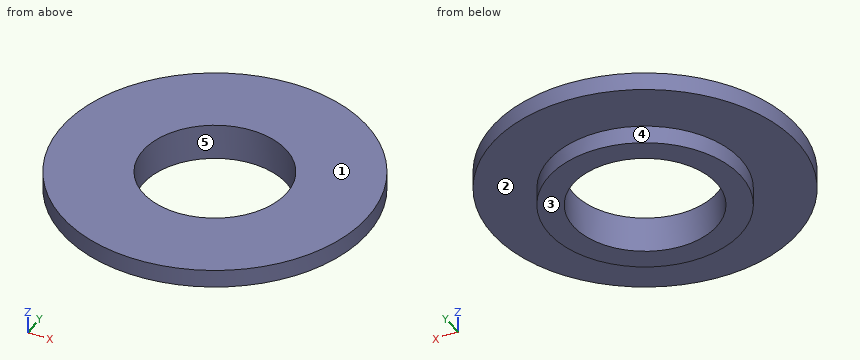
```python
from build123d import *

# Parameters (mm, degrees)
SKETCH_R     = 8.5
PAD_DEPTH    = 1
SKETCH001_R  = 5.35
PAD001_DEPTH = 1
SKETCH002_R  = 4
POCKET_DEPTH = 2.5


with BuildPart() as part:
    # Sketch → Pad (new body)
    with BuildSketch(Plane.XY):
        Circle(SKETCH_R)
    extrude(amount=PAD_DEPTH)

    # Sketch001 → Pad001 (join)
    with BuildSketch(Plane.XY):
        Circle(SKETCH001_R)
    extrude(amount=-PAD001_DEPTH)

    # Sketch002 → Pocket (cut, symmetric)
    with BuildSketch(Plane.XY):
        Circle(SKETCH002_R)
    extrude(amount=POCKET_DEPTH, both=True, mode=Mode.SUBTRACT)


solid = part.part
```
Model file for the job. Use its own axes, mm. Face numbers are marked on the shaded views. A direction names the side the tool comes from. Coordinates: 2 decimals unless noted, no trailing zeros. Order: outer loops, then holes, each group sorted by start corner. A loop starts at its lowest first (then second) coordinate and runs counter-clockwise, first axis right, second up. Notation, with made-up numbers: (-16, -18.5) -> (-10, -18.5) arc R17 ccw to (-10, -9.5) -> close; hole circle Ø8 at (5, -27). An arc over 180 degrees is marked (long way). Answer as a JSON object with one key per item and string values. Group by question number.
1) Cut at D-D, the plane x = -4.5. Write the cut outline in (y, z), then the cut area to 3 significant figures.
2) Pull direction X, two halves, no side cores. Call the marked faces 3, 4 and 5: +X half, -X half, draft (parallel to the pull), parting line (faces both ways), or undercut.
3) Drill centre lines: L1, parallel to Y at x = 0, z = -0.1; L2, parallel to Y at x = 0, z = 0.55; L3, parallel to X at y = -2.75, z = 0.75. Where is each one in solid material? Low to high.
4) Cut at C-C, the plane z = -0.25. Write the cut outline in (x, y).
5) Cut at A-A, the plane x = 0. Write the cut outline in (y, z).
6) Which spindle directions (+Z, -Z, +X, -X, +Y, -Y) get a long thin tool onto all of the face, cutting with end or side? Do the marked faces 1 and 2. Say none if no direction does.
Check values:
{
 "1": {"outline": "(-7.21, 0) -> (-2.89, 0) -> (-2.89, -1) -> (2.89, -1) -> (2.89, 0) -> (7.21, 0) -> (7.21, 1) -> (-7.21, 1) -> close", "area": "20.2 mm²"},
 "2": {"face 3": "draft", "face 4": "parting line", "face 5": "undercut"},
 "3": {"L1": "y = -5.35 to -4, 4 to 5.35", "L2": "y = -8.5 to -4, 4 to 8.5", "L3": "x = -8.04 to -2.9, 2.9 to 8.04"},
 "4": {"outline": "circle Ø10.7 at (0, 0); hole circle Ø8 at (0, 0)"},
 "5": {"outline": "(-8.5, 0) -> (-5.35, 0) -> (-5.35, -1) -> (-4, -1) -> (-4, 1) -> (-8.5, 1) -> close; (4, -1) -> (5.35, -1) -> (5.35, 0) -> (8.5, 0) -> (8.5, 1) -> (4, 1) -> close"},
 "6": {"face 1": "+Z, +X, -X, +Y, -Y", "face 2": "-Z"}
}
